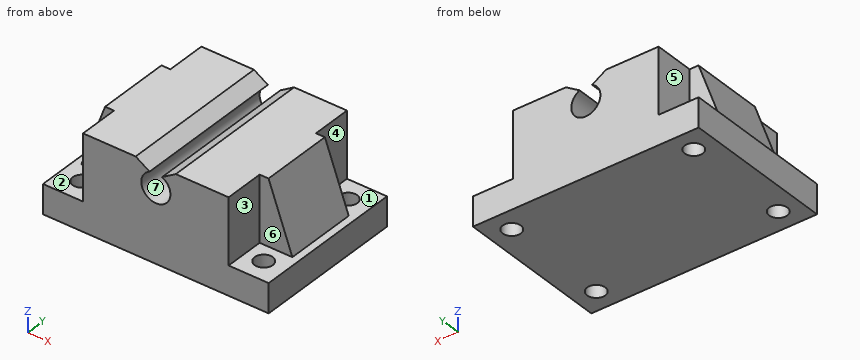
```python
from build123d import *

# Parameters (mm, degrees)
EXTRUDE1_DEPTH        = 21
EXTRUDE1_DEPTH_BACK   = 21
EXTRUDE2_DEPTH        = 10
EXTRUDE2_DEPTH_BACK   = 10
CORTAR_EXTRUIR1_REACH = 28
CROQUIS1_R            = 2.5


with BuildPart() as part:
    # Sketch1 → Extrude1 (new body, two sides)
    with BuildSketch(Plane(origin=(0, 0, 0), x_dir=(1, 0, 0), z_dir=(0, 1, 0))) as extrude1_sk:
        with BuildLine():
            Line((20, -22), (20, -4))
            Line((20, -4), (29, -4))
            Line((29, -4), (31, -4))
            Line((31, -4), (31, 4))
            Line((31, 4), (-31, 4))
            Line((-31, 4), (-31, -4))
            Line((-31, -4), (-29, -4))
            Line((-29, -4), (-20, -4))
            Line((-20, -4), (-20, -22))
            Line((-20, -22), (-5.546820257, -22))
            Line((-5.546820257, -22), (-1.724579107, -19.609131046))
            ThreePointArc((-1.724579107, -19.609131046), (0.008719361, -12.000009503), (1.708828096, -19.616615343))
            Line((1.708828096, -19.616615343), (5.482961188, -22))
            Line((5.482961188, -22), (20, -22))
        make_face()
    extrude(amount=EXTRUDE1_DEPTH)
    extrude(extrude1_sk.sketch, amount=-EXTRUDE1_DEPTH_BACK)

    # Sketch1_8 → Extrude2 (add, two sides)
    with BuildSketch(Plane(origin=(0, 0, 0), x_dir=(1, 0, 0), z_dir=(0, 1, 0))) as extrude2_sk:
        Polygon((29, -4), (20, -4), (20, -22), (22.448535783, -22), align=None)
        Polygon((-20, -4), (-29, -4), (-22.448535783, -22), (-20, -22), align=None)
    extrude(amount=EXTRUDE2_DEPTH)
    extrude(extrude2_sk.sketch, amount=-EXTRUDE2_DEPTH_BACK)

    # Croquis1 → Cortar-Extruir1 (cut, up to next)
    with BuildSketch(Plane(origin=(0, 0, -4), x_dir=(-1, 0, 0), z_dir=(0, 0, -1)), mode=Mode.PRIVATE) as cortar_extruir1_sk1:
        with Locations((-25, 15)):
            Circle(CROQUIS1_R)
    cortar_extruir1_tool1 = extrude(cortar_extruir1_sk1.sketch, amount=-CORTAR_EXTRUIR1_REACH, mode=Mode.PRIVATE) & part.part
    add(cortar_extruir1_tool1.solids().sort_by_distance((25, 15, -4))[0], mode=Mode.SUBTRACT)
    # Croquis1 → Cortar-Extruir1 (cut, up to next)
    with BuildSketch(Plane(origin=(0, 0, -4), x_dir=(-1, 0, 0), z_dir=(0, 0, -1)), mode=Mode.PRIVATE) as cortar_extruir1_sk2:
        with Locations((25, 15)):
            Circle(CROQUIS1_R)
    cortar_extruir1_tool2 = extrude(cortar_extruir1_sk2.sketch, amount=-CORTAR_EXTRUIR1_REACH, mode=Mode.PRIVATE) & part.part
    add(cortar_extruir1_tool2.solids().sort_by_distance((-25, 15, -4))[0], mode=Mode.SUBTRACT)
    # Croquis1 → Cortar-Extruir1 (cut, up to next)
    with BuildSketch(Plane(origin=(0, 0, -4), x_dir=(-1, 0, 0), z_dir=(0, 0, -1)), mode=Mode.PRIVATE) as cortar_extruir1_sk3:
        with Locations((-25, -15)):
            Circle(CROQUIS1_R)
    cortar_extruir1_tool3 = extrude(cortar_extruir1_sk3.sketch, amount=-CORTAR_EXTRUIR1_REACH, mode=Mode.PRIVATE) & part.part
    add(cortar_extruir1_tool3.solids().sort_by_distance((25, -15, -4))[0], mode=Mode.SUBTRACT)
    # Croquis1 → Cortar-Extruir1 (cut, up to next)
    with BuildSketch(Plane(origin=(0, 0, -4), x_dir=(-1, 0, 0), z_dir=(0, 0, -1)), mode=Mode.PRIVATE) as cortar_extruir1_sk4:
        with Locations((25, -15)):
            Circle(CROQUIS1_R)
    cortar_extruir1_tool4 = extrude(cortar_extruir1_sk4.sketch, amount=-CORTAR_EXTRUIR1_REACH, mode=Mode.PRIVATE) & part.part
    add(cortar_extruir1_tool4.solids().sort_by_distance((-25, -15, -4))[0], mode=Mode.SUBTRACT)


solid = part.part
```
The model under review builds one solid part; all positions refer to its coordinate system, in mm. Face numbers are marked on the shaded views. A direction names the side the tool comes from. Round coordinates to 2 decimals unless told otherwise and drop trailing zeros. Loops run counter-clockwise (first coordinate to the right, second up) from the corner with the lowest first, then second, coordinate; pieces in that order, holes last. Notation, with made-up numbers: (46, 12) - (80, 12) arc R30 ccw to (80, 34) - close; hole circle Ø9 at (-1, 37.25). An arc over 180 degrees is marked (long way). Write each question's results on one line, items separated by ' | '. Start each with the question number.
Q1. Insertion check: P1, Ø1, axis at y = -7, z = 10.5, coming from the +X side; P2, Ø8, axis at x = 25, y = 15, coming from the +Z side; P3, Ø2.5, axis at x = -23.5, z = 17, coming from the +Y side. Each pin has a flat end and moves straight along its axis. Give the tip position at first contact, or say it passes through.
Q2. Wall thickness on line 1 along Y through (x, z) = (25, 0.75); line 2 along Y through (x, z) = (-22.5, 13.75); line 3 along X through (y, z) = (2.5, 14): over which ranges is each line inside the solid? List them lowest first. Write a range as [from, to].
Q3. Take a section at D-D on x = -24.5. Give the boundary of the cut face in (y, z), plus the area to 3 significant figures.
Q4. Take a section at C-C on z = 16. Give the boundary of the cut face in (x, y), plus the area to 3 significant figures.
Q5. Tool access review of the marked faces 1, 2 and 3: name each direction out of +Z, -Z, +X, -X, +Y, -Y from which nothing blocks a thin tool from reaching the whole face with its end or side.
Q6. Take a section at A-A on z = -0.75. Give the boundary of the cut face in (x, y), plus the area to 3 significant figures.
Q7. Take a section at B-B on y = 15. Give the boundary of the cut face in (x, z), plus the area to 3 significant figures.
Q8. Draft analysis for pull direction X (two halves, no side actions). For the marked faces 4, 5, 6 and 7, state which applies: pulls with the +X half, pulls with the -X half, needs draft (parallel to the pull), parting line crosses it, or undercut.
Data:
1) P1: stops at x = 26.82 | P2: stops at z = 4 | P3: stops at y = 10
2) line 1: y = [-21, -17.5], [-12.5, 12.5], [17.5, 21] | line 2: y = [-10, 10] | line 3: x = [-25.36, -3.46], [3.46, 25.36]
3) outline: (-21, -4) - (-17.45, -4) - (-17.45, 4) - (-21, 4) - close; (-12.55, -4) - (12.55, -4) - (12.55, 4) - (10, 4) - (10, 16.36) - (-10, 16.36) - (-10, 4) - (-12.55, 4) - close; (17.45, -4) - (21, -4) - (21, 4) - (17.45, 4) - close | area: 505 mm²
4) outline: (-24.63, -10) - (-20, -10) - (-20, -21) - (-4, -21) - (-4, 21) - (-20, 21) - (-20, 10) - (-24.63, 10) - close; (4, -21) - (20, -21) - (20, -10) - (24.63, -10) - (24.63, 10) - (20, 10) - (20, 21) - (4, 21) - close | area: 1,530 mm²
5) face 1: +Z, +X | face 2: +Z, -X | face 3: +Z, +X, -Y
6) outline: (-31, -21) - (31, -21) - (31, 21) - (-31, 21) - close; hole circle Ø5 at (-25, -15); hole circle Ø5 at (-25, 15); hole circle Ø5 at (25, -15); hole circle Ø5 at (25, 15) | area: 2,530 mm²
7) outline: (-31, -4) - (-27.5, -4) - (-27.5, 4) - (-31, 4) - close; (-22.5, -4) - (22.5, -4) - (22.5, 4) - (20, 4) - (20, 22) - (5.48, 22) - (1.71, 19.62) arc R4 cw (long way) to (-1.72, 19.61) - (-5.55, 22) - (-20, 22) - (-20, 4) - (-22.5, 4) - close; (27.5, -4) - (31, -4) - (31, 4) - (27.5, 4) - close | area: 1,070 mm²
8) face 4: pulls with the +X half | face 5: pulls with the -X half | face 6: needs draft | face 7: undercut
